The model under review builds one solid part; all positions refer to its coordinate system, in mm. Coordinates: 2 decimals unless noted, no trailing zeros. Loops run counter-clockwise (first coordinate to the right, second up) from the corner with the lowest first, then second, coordinate; pieces in that order, holes last. Notation, with made-up numbers: (59, 29.5) - (117, 29.5) arc R32 cw to (117, 55.5) - close; hole circle Ø10 at (25, -9). An arc over 180 degrees is marked (long way). Use a Markdown table: item, result. Add a question column.
1) To check wall thickness, follow L1, parallel to Y at x = 40, z = 1.6; L2, parallel to X at y = 50, z = 1.35; L3, parallel to X at y = 44.5, z = 1.45. State the ranges of each line that lie inside material, in increasing order. Write a range as [from, to].
2) Add section A-A, the plane x = 40. Give the boundary of the cut face in (y, z), and give its area (3 significant figures).
3) Add section D-D, the plane z = 1.8. Give the boundary of the cut face in (x, y).
4) Clearance check with flat-ended pins moving along their axes: pin 1 (1 mm diameter, centred on x = 24, y = 11, fed in from -Z); pin 2 (1 mm diameter, centred on y = 31, z = 0.5, fed in from +X). State where each tip first meets the part, or that it passes through.
5) Add section B-B, the plane y = 10. Give the boundary of the cut face in (x, z), and give its area (3 significant figures).
6) Add section C-C, the plane y = 36. Give the boundary of the cut face in (x, z).
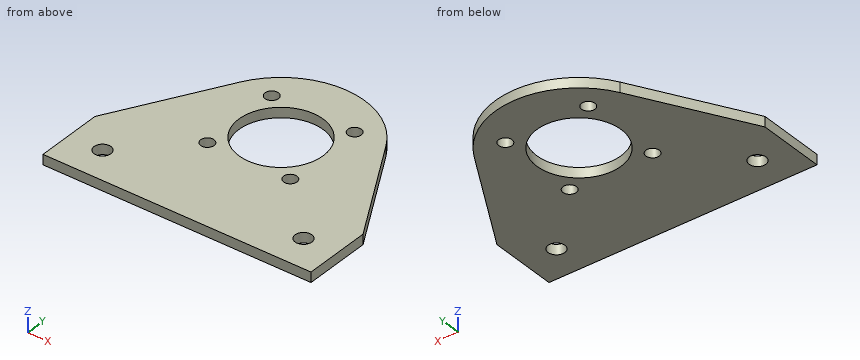
Autodesk Inventor part; units mm, degrees
ref_plane "YZ Plane" through (0, 0, 0) normal (1, 0, 0) x (0, 1, 0)
ref_plane "XZ Plane" through (0, 0, 0) normal (0, 1, 0) x (-1, 0, 0)
ref_plane "XY Plane" through (0, 0, 0) normal (0, 0, 1) x (1, 0, 0)
sketch "スケッチ1" plane through (0, 0, 0) normal (0, 0, 1) x (1, 0, 0)
  line L0 (0, 0) -> (80, 0)
  line L1 (80, 0) -> (80, 20)
  line L2 (40, 0) -> (40, 90.8523) construction
  line L3 (0, 20) -> (0, 0)
  line L4 (0, 20) -> (18.2298, 52.2905)
  line L5 (61.7702, 52.2905) -> (80, 20)
  arc A0 (61.7702, 52.2905) -> (18.2298, 52.2905) centre (40, 40) ccw
  circle A1 centre (40, 40) radius 12.55
  line L6 (0, 10) -> (80, 10) construction
  circle A2 centre (10, 10) radius 2.5
  circle A3 centre (70, 10) radius 2.5
  circle A4 centre (40, 40) radius 17.5 construction
  line L7 (0, 20) -> (80, 20) construction
  line L8 (40, 40) -> (52.3744, 52.3744) construction
  circle A5 centre (52.3744, 52.3744) radius 2
  circle A6 centre (27.6256, 52.3744) radius 2
  circle A7 centre (27.6256, 27.6256) radius 2
  circle A8 centre (52.3744, 27.6256) radius 2
  dimension "d11" = 35
  dimension "d0" = 20
  dimension "d2" = 80
  dimension "d3" = 25
  dimension "d4" = 40
  dimension "d5" = 25.1
  dimension "d6" = 5
  dimension "d7" = 10
  dimension "d17" = 45
  dimension "d18" = 4
  dimension "d21" = 360
extrude "押し出し2" add sketch "スケッチ1" along normal blind 3
properties part number "車軸受け板"
From the geometry:
| question | item | result |
|---|---|---|
| 1 | L1 | y = [0, 27.45], [52.55, 65] |
| 1 | L2 | x = [16.94, 32.42], [47.58, 63.06] |
| 1 | L3 | x = [13.83, 28.28], [51.72, 66.17] |
| 2 | outline | (0, 0) - (27.45, 0) - (27.45, 3) - (0, 3) - close; (52.55, 0) - (65, 0) - (65, 3) - (52.55, 3) - close |
| 2 | area | 120 mm^2 |
| 3 | outline | (0, 0) - (80, 0) - (80, 20) - (61.77, 52.29) arc R25 ccw to (18.23, 52.29) - (0, 20) - close; hole circle Ø5 at (10, 10); hole circle Ø4 at (27.63, 27.63); hole circle Ø4 at (27.63, 52.37); hole circle Ø25.1 at (40, 40); hole circle Ø4 at (52.37, 27.63); hole circle Ø4 at (52.37, 52.37); hole circle Ø5 at (70, 10) |
| 4 | pin 1 | stops at z = 0 |
| 4 | pin 2 | stops at x = 74.07 |
| 5 | outline | (0, 0) - (7.5, 0) - (7.5, 3) - (0, 3) - close; (12.5, 0) - (67.5, 0) - (67.5, 3) - (12.5, 3) - close; (72.5, 0) - (80, 0) - (80, 3) - (72.5, 3) - close |
| 5 | area | 210 mm^2 |
| 6 | outline | (9.03, 0) - (28.1, 0) - (28.1, 3) - (9.03, 3) - close; (51.9, 0) - (70.97, 0) - (70.97, 3) - (51.9, 3) - close |
